from build123d import *

# Parameters (mm, degrees)
SKETCH_1_W          = 20
SKETCH_1_H          = 12
EXTRUDE_1_DEPTH     = 0.8
FILLET_2_R          = 0.4
SKETCH_2_W          = 1.91
SKETCH_2_H          = 1.11
CUT_EXTRUDE_1_DEPTH = 14.307269619


with BuildPart() as part:
    # 草图1 → 凸台-拉伸1 (new body)
    with BuildSketch(Plane.XY):
        with Locations((0.967032967, -1.494505495)):
            Rectangle(SKETCH_1_W, SKETCH_1_H)
    extrude(amount=EXTRUDE_1_DEPTH)

    # 圆角2
    fillet_2_edges = [part.edges().sort_by_distance(p)[0] for p in [
        (10.967032967, -1.494505495, 0.8),
        (0.967032967, 4.505494505, 0.8),
        (-9.032967033, -1.494505495, 0.8),
        (0.967032967, 4.505494505, 0),
        (10.967032967, -1.494505495, 0),
        (0.967032967, -7.494505495, 0),
        (-9.032967033, -1.494505495, 0),
        (0.967032967, -7.494505495, 0.8),
        (-9.032967033, 4.505494505, 0.4),
        (10.967032967, 4.505494505, 0.4),
        (10.967032967, -7.494505495, 0.4),
        (-9.032967033, -7.494505495, 0.4),
    ]]
    fillet(fillet_2_edges, radius=FILLET_2_R - 0.0001)  # a hair under: the kernel refuses the full size

    # 草图2 → 切除-拉伸1 (cut, through all)
    with BuildSketch(Plane(origin=(0, 0, 0), x_dir=(-1, 0, 0), z_dir=(0, 0, -1))):
        with Locations((-7.212032967, 2.600494505)):
            Rectangle(SKETCH_2_W, SKETCH_2_H)
        with Locations((-7.212032967, -5.589505495)):
            Rectangle(SKETCH_2_W, SKETCH_2_H)
        with Locations((5.277967033, 2.600494505)):
            Rectangle(SKETCH_2_W, SKETCH_2_H)
        with Locations((5.277967033, -5.589505495)):
            Rectangle(SKETCH_2_W, SKETCH_2_H)
    extrude(amount=-CUT_EXTRUDE_1_DEPTH, mode=Mode.SUBTRACT)


solid = part.part
For this review, take the finished solid that the model builds, in its own axes (mm). Round coordinates to 2 decimals unless told otherwise and drop trailing zeros. Loops run counter-clockwise (first coordinate to the right, second up) from the corner with the lowest first, then second, coordinate; pieces in that order, holes last. Notation, with made-up numbers: (43, -25.75) - (78, -25.75) arc R21 cw to (78, 8.25) - close; hole circle Ø10 at (-27.75, -21.75). An arc over 180 degrees is marked (long way). Use one line per item in the form item = value.
Item 1: For line 1 (Y direction, x = -4.5, z = 0.2); line 2 (Y direction, x = 8, z = 0.3); line 3 (X direction, y = -2.25, z = 0.45), list the stretches that pass through material, from the lowest coordinate up.
Answers:
line_1 = -7.44 to -6.14, -5.03 to 2.05, 3.16 to 4.45
line_2 = -7.48 to -6.14, -5.03 to 2.05, 3.16 to 4.49
line_3 = -9.03 to 10.96
Item 2: Consider section B-B on z = 0.65. Write out the cut boundary in (x, y), then the cut area to 3 significant figures.
Answers:
outline = (-8.95, -7.09) arc R0.31 ccw to (-8.63, -7.41) - (10.57, -7.41) arc R0.31 ccw to (10.88, -7.09) - (10.88, 4.11) arc R0.31 ccw to (10.57, 4.42) - (-8.63, 4.42) arc R0.31 ccw to (-8.95, 4.11) - close; hole (-6.23, -6.14) - (-4.32, -6.14) - (-4.32, -5.03) - (-6.23, -5.03) - close; hole (-6.23, 2.05) - (-4.32, 2.05) - (-4.32, 3.16) - (-6.23, 3.16) - close; hole (6.26, -6.14) - (8.17, -6.14) - (8.17, -5.03) - (6.26, -5.03) - close; hole (6.26, 2.05) - (8.17, 2.05) - (8.17, 3.16) - (6.26, 3.16) - close
area = 226 mm^2
Item 3: Consider section A-A on x = -5.75. State how many separate pieces and enclosed holes the cut face has, then the cut area to 3 significant figures.
Answers:
separate_pieces = 3
enclosed_holes = 0
area = 7.69 mm^2
